```python
from build123d import *

# Parameters (mm, degrees)
F0_R     = 8.75
F1_DEPTH = 60
F2_DEPTH = 10
F3_SIZE  = 5


with BuildPart() as f1:
    # F0 (on Top) → F1 (new body)
    with BuildSketch(Plane.XY):
        Circle(F0_R)
    extrude(amount=-F1_DEPTH)

    # F0 (on Top) → F2 (join)
    with BuildSketch(Plane.XY):
        Polygon((13.656054, -7.884326), (13.656054, 7.884326), (0, 15.768653), (-13.656054, 7.884326), (-13.656054, -7.884326), (0, -15.768653), align=None)
        Circle(F0_R, mode=Mode.SUBTRACT)
        Circle(F0_R)
    extrude(amount=-F2_DEPTH)

    # F3
    f3_edges = [f1.edges().sort_by_distance(p)[0] for p in [
        (-8.75, 0, -60),
    ]]
    chamfer(f3_edges, length=F3_SIZE)


solid = f1.part
```
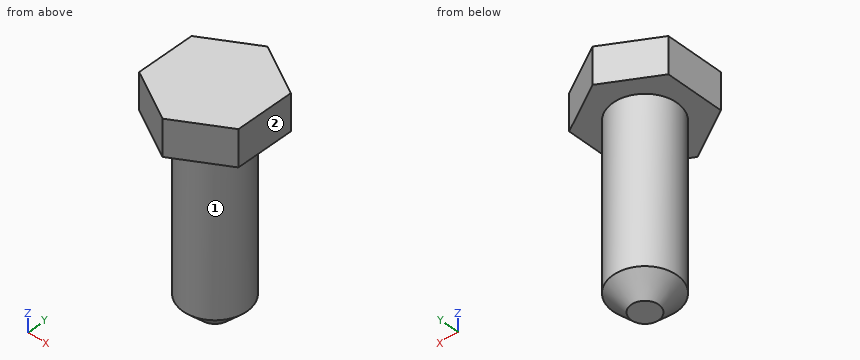
Could you check a few things on this model? Use its own coordinates, in mm. Face numbers are marked on the shaded views. A direction names the side the tool comes from. Give positions to 0.01 mm unless a question says otherwise; leave off trailing zeros. Order: outer loops, then holes, each group sorted by start corner. A loop starts at its lowest first (then second) coordinate and runs counter-clockwise, first axis right, second up.
Q1. Suppose I cut it at A-A, the plane y = 0. Write out the boundary of the cut face in (x, z), and give its area (3 significant figures).
Q2. I'm going to push flat-ended pins straight in: P1, Ø3, axis at x = -10.5, z = -13.5, coming from the -Y side; P2, Ø1.5, axis at y = 0, z = -41, coming from the +X side; P3, Ø12, axis at x = 0.5, y = 1.5, coming from the +Z side; P4, Ø1.5, axis at y = -8, z = -38.5, coming from the +X side. Where does each tip first touch, or does it pass through?
Q3. Suppose I cut it at C-C, the plane z = -48. Write out the boundary of the cut face in (x, y), and give its area (3 significant figures).
Q4. If I drill on line 1 along Z through (x, y) = (12.5, 7); line 2 along X through (y, z) = (11, -5); line 3 along Y through (x, z) = (1.5, -47), over which ranges is the centre line in solid material (lowest first)?
Q5. Suppose I cut it at D-D, the plane y = 12.5. Write out the boundary of the cut face in (x, z).
Q6. Suppose I cut it at B-B, the plane z = -6. Write out the boundary of the cut face in (x, y).
Q7. For the marked faces 1 and 2, which set-ups out of +Z, -Z, +X, -X, +Y, -Y let a thin tool reach every point of the face, with its end or its side?
Solution:
1. outline: (-13.66, -10) - (-8.75, -10) - (-8.75, -55) - (-3.75, -60) - (3.75, -60) - (8.75, -55) - (8.75, -10) - (13.66, -10) - (13.66, 0) - (-13.66, 0) - close
1. area: 1,120 mm2
2. P1: passes through
2. P2: stops at x = 8.75
2. P3: stops at z = 0
2. P4: stops at x = 4.9
3. outline: circle Ø17.5 at (0, 0)
3. area: 241 mm2
4. line 1: z = -10 to 0
4. line 2: x = -8.26 to 8.26
4. line 3: y = -8.62 to 8.62
5. outline: (-5.66, -10) - (5.66, -10) - (5.66, 0) - (-5.66, 0) - close
6. outline: (-13.66, -7.88) - (0, -15.77) - (13.66, -7.88) - (13.66, 7.88) - (0, 15.77) - (-13.66, 7.88) - close
7. face 1: -Z
7. face 2: +Z, -Z, +X, +Y, -Y
